from build123d import *

# Parameters (mm, degrees)
BOSS_EXTRUDE1_DEPTH = 853.44
SKETCH2_R           = 11.1125
CUT_EXTRUDE1_DEPTH  = 25.4
LPATTERN1_COUNT     = 12
LPATTERN1_PITCH     = 44.45
SKETCH3_R           = 7.9375
CUT_EXTRUDE2_DEPTH  = 25.4
SKETCH5_R           = 1.5875
CUT_EXTRUDE3_DEPTH  = 12.7


with BuildPart() as part:
    # Sketch1 → Boss-Extrude1 (new body)
    with BuildSketch(Plane.XY):
        with BuildLine():
            Line((-13.154409933, 15.906683314), (-8.074409933, 15.906683314))
            ThreePointArc((-8.074409933, 15.906683314), (0.597692516, 19.498785762), (-2.994409933, 10.826683314))
            Line((-2.994409933, 10.826683314), (-8.074409933, 10.826683314))
            Line((-8.074409933, 10.826683314), (-8.074409933, -19.018316686))
            Line((-8.074409933, -19.018316686), (-2.994409933, -19.018316686))
            ThreePointArc((-2.994409933, -19.018316686), (0.597692516, -27.690419135), (-8.074409933, -24.098316686))
            Line((-8.074409933, -24.098316686), (-13.154409933, -24.098316686))
            Line((-13.154409933, -24.098316686), (-13.154409933, 15.906683314))
        make_face()
    extrude(amount=BOSS_EXTRUDE1_DEPTH)

    # Sketch2 → Cut-Extrude1 (cut)
    with BuildSketch(Plane.ZY.offset(13.154409933)):
        with Locations(Location((152.4, -4.095816686, 0), (0, 0, 270))):
            Circle(SKETCH2_R)
    cut_extrude1 = extrude(amount=-CUT_EXTRUDE1_DEPTH, mode=Mode.SUBTRACT)

    # LPattern1: Cut-Extrude1 ×12
    with Locations(*[(0, 0, i * LPATTERN1_PITCH) for i in range(1, LPATTERN1_COUNT)]):
        add(cut_extrude1, mode=Mode.SUBTRACT)

    # Sketch3 → Cut-Extrude2 (cut)
    with BuildSketch(Plane.ZY.offset(13.154409933)):
        with Locations(Location((834.39, -4.095816686, 0), (0, 0, 270))):
            Circle(SKETCH3_R)
        with BuildLine():
            Line((31.75, 3.841683314), (57.15, 3.841683314))
            ThreePointArc((57.15, 3.841683314), (65.0875, -4.095816686), (57.15, -12.033316686))
            Line((57.15, -12.033316686), (31.75, -12.033316686))
            ThreePointArc((31.75, -12.033316686), (23.8125, -4.095816686), (31.75, 3.841683314))
        make_face()
    extrude(amount=-CUT_EXTRUDE2_DEPTH, mode=Mode.SUBTRACT)

    # Sketch5 → Cut-Extrude3 (cut)
    with BuildSketch(Plane.ZY.offset(13.154409933)):
        with Locations(Location((734.568, 8.794683314, 0), (0, 0, 270))):
            Circle(SKETCH5_R)
        with Locations(Location((808.228, 8.794683314, 0), (0, 0, 270))):
            Circle(SKETCH5_R)
        with Locations(Location((803.148, -16.986316686, 0), (0, 0, 270))):
            Circle(SKETCH5_R)
        with Locations(Location((734.568, -16.986316686, 0), (0, 0, 270))):
            Circle(SKETCH5_R)
    extrude(amount=-CUT_EXTRUDE3_DEPTH, mode=Mode.SUBTRACT)


solid = part.part
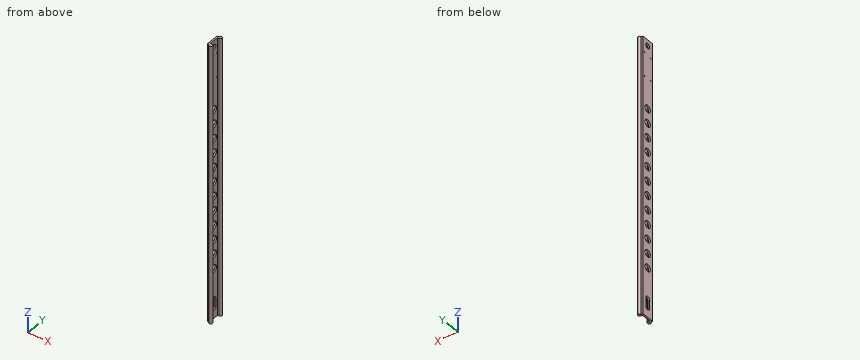
For this review, take the finished solid that the model builds, in its own axes (mm). Give positions to 0.01 mm unless a question says otherwise; leave off trailing zeros. Loops run counter-clockwise (first coordinate to the right, second up) from the corner with the lowest first, then second, coordinate; pieces in that order, holes last. Notation, with made-up numbers: M 57.5,-17.5 L 91.5,-17.5 A18 ccw 91.5,8.5 Z; hole C -33,0 d3. An arc over 180 degrees is marked long. Answer as a JSON object with one key per item and string values. Group by question number.
Q1. Add section B-B on z = 330.2. Give the boundary of the cut face in (x, y).
Q2. Add section A-A on z = 834.39. Give the boundary of the cut face in (x, y).
Q3. Insertion check: P1, Ø1, axis at x = -7, y = -1, coming from the -Z side (3 decimals); P2, Ø3, axis at x = -10, z = 337.5, coming from the +Y side; P3, Ø8, axis at x = -6, y = 2, coming from the +Z side; P4, Ø1, axis at x = -10, z = 646, coming from the -Y side. Each pin has a flat end and moves straight along its axis. Give the tip position at first contact, or say it passes through.
Q4. For probe 1 along Y at (x, z) = (-11.9, 834.39); probe 2 along Y at (x, z) = (-2, 422); probe 3 along X at (y, z) = (7.5, 44.5), list the stretches that pass through material, from the lowest coordinate up. Write a range as [from, to].
Checked values:
{
 "1": {"outline": "M -13.15,-24.1 L -8.07,-24.1 A5.08 ccw long -2.99,-19.02 L -8.07,-19.02 L -8.07,-15.21 L -13.15,-15.21 Z; M -13.15,7.02 L -8.07,7.02 L -8.07,10.83 L -2.99,10.83 A5.08 ccw long -8.07,15.91 L -13.15,15.91 Z"},
 "2": {"outline": "M -13.15,-24.1 L -8.07,-24.1 A5.08 ccw long -2.99,-19.02 L -8.07,-19.02 L -8.07,-12.03 L -13.15,-12.03 Z; M -13.15,3.84 L -8.07,3.84 L -8.07,10.83 L -2.99,10.83 A5.08 ccw long -8.07,15.91 L -13.15,15.91 Z"},
 "3": {"P1": "through", "P2": "y = 15.91", "P3": "z = 853.44", "P4": "y = -24.1"},
 "4": {"probe 1": "[-24.1, -12.03], [3.84, 15.91]", "probe 2": "[-29.08, -19.12], [10.92, 20.89]", "probe 3": "[-13.15, -8.07]"}
}
